```python
from build123d import *

# Parameters (mm, degrees)
BOSS_EXTRUDE1_DEPTH = 2.9972
EXTRUDE_THIN1_REACH = 270.741
FILLET1_R           = 17.78


with BuildPart() as part:
    # Sketch1 → Boss-Extrude1 (new body)
    with BuildSketch(Plane.XY):
        Polygon((0, 0), (177.3936, 88.9), (253.5936, 88.9), (203.2, 0), (127, 0), (127, -12.7), (76.9874, -12.7), (76.9874, 0), align=None)
    extrude(amount=BOSS_EXTRUDE1_DEPTH)

    # Extrude-Thin1: up to this plane
    extrude_thin1_end = Plane(origin=(253.5936, 88.9, 2.9972), z_dir=(-0.8699511006630548, 0.4931379953472858, 0))
    # Sketch2 → Extrude-Thin1 (add, up to the surface)
    with BuildSketch(Plane(origin=(0, 0, 0), x_dir=(0, 0, -1), z_dir=(1, 0, 0)), mode=Mode.PRIVATE) as extrude_thin1_sk1:
        with BuildLine():
            ThreePointArc((-14.1986, -1.591002342), (-1.4986, 0.022109161), (11.2014, -1.591002342))
            Line((11.2014, -1.591002342), (11.200765, -1.593461686))
            ThreePointArc((11.200765, -1.593461686), (-1.4986, 0.019569161), (-14.197965, -1.593461686))
            Line((-14.197965, -1.593461686), (-14.1986, -1.591002342))
        make_face()
    extrude_thin1_tool1 = split(extrude(extrude_thin1_sk1.sketch, amount=EXTRUDE_THIN1_REACH, mode=Mode.PRIVATE), bisect_by=extrude_thin1_end, keep=Keep.BOTH, mode=Mode.PRIVATE)
    add(extrude_thin1_tool1.solids().sort_by_distance((0, -1.528604, -10.954651))[0])

    # Fillet1
    # the kernel refuses this fillet: 17.78 mm, written as the material it adds along each edge
    with BuildSketch(Plane(origin=(0, 0, 0), x_dir=(0, -0.1406246122093386, -0.9900629871078774), z_dir=(1, 0, 0))) as fillet1_piece_1_section:
        with BuildLine():
            CenterArc((15.504190696, 17.279156247), FILLET1_R, 188.083991465, 68.284382717)
            Line((-2.099129215, 14.778850642), (0, 0))
            ThreePointArc((0, 0), (5.656912816, 0.315949673), (11.313825631, 0))
        make_face()
    fillet1_piece_1 = extrude(amount=240.517955612, mode=Mode.PRIVATE)
    fillet1_piece_1 = split(fillet1_piece_1, bisect_by=Plane(origin=(86.561023995, 43.379665519, -3.035000441), z_dir=(0.4480326676326847, -0.89401718592762, 0)), keep=Keep.TOP, mode=Mode.PRIVATE)
    fillet1_piece_1 = split(fillet1_piece_1, bisect_by=Plane(origin=(181.635497998, -38.042216233, -3.035000441), z_dir=(-0.8699511006630548, 0.4931379953472858, 0)), keep=Keep.TOP, mode=Mode.PRIVATE)
    add(fillet1_piece_1)
    with BuildSketch(Plane(origin=(240.517955612, 0, 2.9972), x_dir=(0, 1, 0), z_dir=(-1, 0, 0))) as fillet1_piece_2_section:
        with BuildLine():
            CenterArc((14.927182245, -17.78), FILLET1_R, 90, 68.284382717)
            ThreePointArc((-1.591002342, -11.2014), (-0.482691094, -5.6451303), (0, 0))
            Line((0, 0), (14.927182245, 0))
        make_face()
    fillet1_piece_2 = extrude(amount=240.517955612, mode=Mode.PRIVATE)
    fillet1_piece_2 = split(fillet1_piece_2, bisect_by=Plane(origin=(86.561023995, 43.379665519, 6.032200441), z_dir=(0.4480326676326847, -0.89401718592762, 0)), keep=Keep.TOP, mode=Mode.PRIVATE)
    fillet1_piece_2 = split(fillet1_piece_2, bisect_by=Plane(origin=(181.635497998, -38.042216233, 6.032200441), z_dir=(-0.8699511006630548, 0.4931379953472858, 0)), keep=Keep.TOP, mode=Mode.PRIVATE)
    add(fillet1_piece_2)


solid = part.part
```
CAD build for the part. Positions are in the model's coordinates, mm. A direction names the side the tool comes from. Coordinates: 2 decimals unless noted, no trailing zeros. Order: outer loops, then holes, each group sorted by start corner. A loop starts at its lowest first (then second) coordinate and runs counter-clockwise, first axis right, second up. Notation, with made-up numbers: (76.25, 89) -> (130.25, 89) arc R25 ccw to (130.25, 127) -> close; hole circle Ø6 at (33.25, 18). An arc over 180 degrees is marked (long way). Use one line per item in the form item = value. Start each with the question number.
1) Tool access for faces 5 (the flat face through (75.97, 38.07, 1.45)), 6 (the flat face through (168, 44, 0)), 7 (the flat face through (168, 44, 2.997)): list every direction of +Z, -Z, +X, -X, +Y, -Y with a clear straight run to the whole face (end or side of a thin tool).
2) Drill centre lines: L1, parallel to Z at x = 149.5, y = 33.5; L2, parallel to Y at x = 158.5, z = 6.5; L3, parallel to Y at x = 201, z = -4.75. Where is each one in solid material? Low to high. Write a range as [from, to].
3) Drop flat-ended pins along their axis: pin 1 (1 mm diameter, centred on y = 4, z = -3, fed in from +X); pin 2 (6.5 mm diameter, centred on x = 109.5, y = -7.5, fed in from -Z); pin 3 (1 mm diameter, centred on x = 174, z = 8.5, fed in from +Y). Give the stop position or say it passes through.
4) Band-saw the part on C-C on y = 35.5. Give the cut face in (x, z), then the cut area to 3 significant figures.
5) Band-saw the part on B-B on z = 7. Give the cut face in (x, y).
6) Pull direction Z, two halves, no side cores. Call faces 1 (the cylindrical face through (100.18, -0.47, 8.52)), 2 (the flat face through (222.365, 33.81, 1.558)), 3 (the cylindrical face through (104.349, 5.071, -2.982)), 4 (the cylindrical face through (100.18, -0.49, -5.68)): +Z half, -Z half, draft (parallel to the pull), parting line (faces both ways), or undercut.
Entries:
q1.face_5 = +Z, -Z, -X, +Y
q1.face_6 = -Z, +X, -X, +Y
q1.face_7 = +Z, +X, -X, +Y
q2.L1 = [0, 3]
q2.L2 = [-0.23, 4.33]
q2.L3 = [-0.37, 2.83]
q3.pin_1 = 205.75
q3.pin_2 = 0
q3.pin_3 = 2.56
q4.outline = (70.84, 0) -> (223.32, 0) -> (223.32, 3) -> (70.84, 3) -> close
q4.area = 457 mm2
q5.outline = (0, -0.28) -> (203.04, -0.28) -> (205.29, 3.69) -> (7.36, 3.69) -> (0, 0) -> close
q6.face_1 = undercut
q6.face_2 = draft
q6.face_3 = -Z half
q6.face_4 = undercut
